Can you work these out from the model? Positions are in its coordinate system, mm. A direction names the side the tool comes from. Give positions to 0.01 mm unless a question says otherwise; leave off trailing zeros. Order: outer loops, then holes, each group sorted by start corner. A loop starts at its lowest first (then second) coordinate and runs counter-clockwise, first axis right, second up. Notation, with made-up numbers: M 50,63 L 54,63 A11 ccw 54,78 Z; hole C 2,50.25 d3. An arc over 180 degrees is marked long. One line per question, with ' | ' between items. Start each with the question number.
1) If we section it at B-B, the plane z = 7.5: Please give me the cut outline in (x, y).
2) Please list where these lines run through material, in increasing order: line 1 along Z through (x, y) = (1.05, 2); line 2 along Y through (x, z) = (1.95, 3); line 3 along X through (y, z) = (-1.2, 12.75). Write a range as [from, to].
3) Thinking about a two-plate mould opening in Z: for faces 3 (the cylindrical face through (-1.62, 1.49, 17.75)), 4 (the flat face through (0, 0, 0)), 5 (the cylindrical face through (-0.54, -2.44, 11.16)), which applies, +Z half, -Z half, draft (parallel to the pull), parting line (faces both ways), or undercut?
4) I'm going to push flat-ended pins straight in: pin 1 Ø2 at (x, z) = (-2, 4) entering from +Y; pin 2 Ø2 at (x, z) = (-1.5, 7.5) entering from +Y; pin 3 Ø2 at (y, z) = (1.5, 12.5) entering from +X. Where does each tip first touch, or does it pass through?
5) If we section it at A-A, the plane x = 1.45: Please give me the cut outline in (y, z).
6) If we section it at C-C, the plane y = -1.25: Please give me the cut outline in (x, z).
7) For faces 1 (the flat face through (0, 0, 23)), 2 (the cylindrical face through (-2.1, 0.66, 4.75)), which set-ups out of +Z, -Z, +X, -X, +Y, -Y let a thin tool reach every point of the face, with its end or its side?
```python
from build123d import *

# Parameters (mm, degrees)
SKETCH1_R                  = 2.5
BOSS_EXTRUDE1_DEPTH        = 23
WYTNIJ_WYCI_GNI_CIE1_START = -5
SZKIC1_R                   = 2.5
SZKIC1_R_2                 = 2.201367386
WYTNIJ_WYCI_GNI_CIE1_DEPTH = 0.5
WYTNIJ_WYCI_GNI_CIE2_START = -5
SZKIC2_R                   = 2.5
SZKIC2_R_2                 = 2.2
WYTNIJ_WYCI_GNI_CIE2_DEPTH = 0.5


with BuildPart() as part:
    # Sketch1 → Boss-Extrude1 (new body)
    with BuildSketch(Plane.XY):
        Circle(SKETCH1_R)
    extrude(amount=BOSS_EXTRUDE1_DEPTH)

    # Szkic1 → Wytnij-wyciągnięcie1 (cut)
    with BuildSketch(Plane.XY.offset(23).offset(WYTNIJ_WYCI_GNI_CIE1_START)):
        Circle(SZKIC1_R)
        Circle(SZKIC1_R_2, mode=Mode.SUBTRACT)
    extrude(amount=-WYTNIJ_WYCI_GNI_CIE1_DEPTH, mode=Mode.SUBTRACT)

    # Szkic2 → Wytnij-wyciągnięcie2 (cut)
    with BuildSketch(Plane(origin=(0, 0, 0), x_dir=(-1, 0, 0), z_dir=(0, 0, -1)).offset(WYTNIJ_WYCI_GNI_CIE2_START)):
        Circle(SZKIC2_R)
        Circle(SZKIC2_R_2, mode=Mode.SUBTRACT)
    extrude(amount=WYTNIJ_WYCI_GNI_CIE2_DEPTH, mode=Mode.SUBTRACT)


solid = part.part
```
Results found:
1) outline: C 0,0 d5
2) line 1: z = [0, 4.5], [5, 17.5], [18, 23] | line 2: y = [-1.56, 1.56] | line 3: x = [-2.19, 2.19]
3) face 3: undercut | face 4: -Z half | face 5: draft
4) pin 1: stops at y = 2.29 | pin 2: stops at y = 2.45 | pin 3: stops at x = 2.45
5) outline: M -2.04,0 L 2.04,0 L 2.04,4.5 L 1.65,4.5 L 1.65,5 L 2.04,5 L 2.04,17.5 L 1.66,17.5 L 1.66,18 L 2.04,18 L 2.04,23 L -2.04,23 L -2.04,18 L -1.66,18 L -1.66,17.5 L -2.04,17.5 L -2.04,5 L -1.65,5 L -1.65,4.5 L -2.04,4.5 Z
6) outline: M -2.17,0 L 2.17,0 L 2.17,4.5 L 1.81,4.5 L 1.81,5 L 2.17,5 L 2.17,17.5 L 1.81,17.5 L 1.81,18 L 2.17,18 L 2.17,23 L -2.17,23 L -2.17,18 L -1.81,18 L -1.81,17.5 L -2.17,17.5 L -2.17,5 L -1.81,5 L -1.81,4.5 L -2.17,4.5 Z
7) face 1: +Z, +X, -X, +Y, -Y | face 2: none
